from build123d import *

# Parameters (mm, degrees)
SKETCH2_R           = 2.168725958
SKETCH2_R_2         = 2.299626563
SKETCH2_R_3         = 2.061813599
SKETCH2_R_4         = 2.159
BOSS_EXTRUDE1_DEPTH = 2.54
SKETCH3_W           = 2.54
SKETCH3_H           = 88.215633797
BOSS_EXTRUDE2_DEPTH = 17.78
SKETCH5_R           = 3.175
CUT_EXTRUDE2_DEPTH  = 17.78


with BuildPart() as part:
    # Sketch2 → Boss-Extrude1 (new body)
    with BuildSketch(Plane.XY):
        Polygon((33.041228817, 37.6809), (33.041228817, 9.671924958), (33.041228817, -38.409527683), (33.041228817, -46.223073917), (-33.041228817, -46.223073917), (-33.041228817, -38.409527683), (-33.041228817, 9.671924958), (-33.041228817, 37.6809), (-33.041228817, 41.99255988), (33.041228817, 41.99255988), align=None)
        with Locations((19.8374, -24.8158)):
            Circle(SKETCH2_R, mode=Mode.SUBTRACT)
        with Locations((21.996003552, 27.558503658)):
            Circle(SKETCH2_R, mode=Mode.SUBTRACT)
        with Locations((-0.000312071, 34.695463786)):
            Circle(SKETCH2_R_2, mode=Mode.SUBTRACT)
        with Locations((-21.9964, 27.559)):
            Circle(SKETCH2_R_3, mode=Mode.SUBTRACT)
        with Locations((-19.8374, 14.859)):
            Circle(SKETCH2_R_4, mode=Mode.SUBTRACT)
        with Locations((-19.8374, -24.8158)):
            Circle(SKETCH2_R, mode=Mode.SUBTRACT)
        Polygon((15.652792396, 9.671924958), (15.652792396, 27.558503658), (-13.85744492, 27.558503658), (-15.780925581, 27.558503658), (-15.780925581, 9.671924958), (-15.780925581, -38.409527683), (15.652792396, -38.409527683), align=None, mode=Mode.SUBTRACT)
    extrude(amount=BOSS_EXTRUDE1_DEPTH)

    # Sketch3 → Boss-Extrude2 (add)
    with BuildSketch(Plane.XY.offset(2.54)):
        with Locations((-31.771228817, -2.115257018)):
            Rectangle(SKETCH3_W, SKETCH3_H)
    extrude(amount=BOSS_EXTRUDE2_DEPTH)

    # Sketch5 → Cut-Extrude2 (cut)
    with BuildSketch(Plane(origin=(-30.501228817, 0, 0), x_dir=(0, 0, -1), z_dir=(1, 0, 0))):
        with Locations((-11.43, -35.196119692)):
            Circle(SKETCH5_R)
        with Locations((-11.43, -13.142211243)):
            Circle(SKETCH5_R)
        with Locations((-11.43, 8.911697206)):
            Circle(SKETCH5_R)
        with Locations((-11.43, 30.965605655)):
            Circle(SKETCH5_R)
    extrude(amount=-CUT_EXTRUDE2_DEPTH, mode=Mode.SUBTRACT)


solid = part.part
Source: CAD feature listing. Evaluate the final solid. Frame: model axes, mm. A direction names the side the tool comes from. Give positions to 0.01 mm unless a question says otherwise; leave off trailing zeros. Write each loop counter-clockwise with the first axis right and the second up, starting at its lowest first coordinate (ties: lowest second). Pieces come first, ordered by that corner, then holes. Notation, with made-up numbers: (31.5, 41) -> (54.5, 41) arc R13 ccw to (54.5, 66) -> close; hole circle Ø11 at (8, 85.25). An arc over 180 degrees is marked (long way). Return JSON: item names as keys, results as strings. Group by question number.
1. Material intervals for line 1 (Y direction, x = -31.35, z = 11.43); line 2 (Y direction, x = 20, z = 2.25); line 3 (X direction, y = 25, z = 1.5), sorted ascending. Write a range as from..to.
2. Section C-C, the plane z = 11.43. Output: boundary loops of the cut face in (x, y).
3. Access query for faces 1 (the face through (33.041, -3, 1)), 2 (the face through (0, 27.559, 1)), 3 (the face through (16, -1, 2.54)). Directions: +Z, -Z, +X, -X, +Y, -Y. A direction counts if a zero-diameter tool reaches every point of the face in a straight line with its end or side. Return the directions, or none.
4. Section B-B, the plane x = -7.5. Output: boundary loops of the cut face in (y, z), then the cut area to 3 significant figures.
5. Section D-D, the plane x = 27. Output: boundary loops of the cut face in (y, z), then the cut area to 3 significant figures.
6. Mould query, pull axis Y, two halves, no side actions, for faces 4 (the face through (-33.041, -3, 10)), 5 (the face through (21.53, 25.44, 1.25)), 6 (the face through (-7, 41.993, 2)). Classes: +Y half, -Y half, draft (parallel to the pull), parting line (faces both ways), or undercut.
7. Section A-A, the plane y = 22. Output: boundary loops of the cut face in (x, z).
8. Pin query (flat end, axial travel): pin 1 Ø7.5 at (x, y) = (0, 34.7) entering from -Z; pin 2 Ø4 at (x, y) = (-19.84, -24.82) entering from -Z; pin 3 Ø2 at (x, y) = (22, -22.5) entering from +Z; pin 4 Ø7.5 at (y, z) = (8.91, 11.43) entering from +X. Return the tip coordinate at first contact, or that it passes through.
Determined:
{
 "1": {"line 1": "y = -46.22..-38.37, -32.02..-16.32, -9.97..5.74, 12.09..27.79, 34.14..41.99", "line 2": "y = -46.22..-26.98, -22.65..26.71, 28.41..41.99", "line 3": "x = -33.04..-15.78, 15.65..33.04"},
 "2": {"outline": "(-33.04, -46.22) -> (-30.5, -46.22) -> (-30.5, -38.37) -> (-33.04, -38.37) -> close; (-33.04, -32.02) -> (-30.5, -32.02) -> (-30.5, -16.32) -> (-33.04, -16.32) -> close; (-33.04, -9.97) -> (-30.5, -9.97) -> (-30.5, 5.74) -> (-33.04, 5.74) -> close; (-33.04, 12.09) -> (-30.5, 12.09) -> (-30.5, 27.79) -> (-33.04, 27.79) -> close; (-33.04, 34.14) -> (-30.5, 34.14) -> (-30.5, 41.99) -> (-33.04, 41.99) -> close"},
 "3": {"face 1": "+Z, -Z, +X, +Y, -Y", "face 2": "+Z, -Z", "face 3": "+Z, +X, +Y, -Y"},
 "4": {"outline": "(-46.22, 0) -> (-38.41, 0) -> (-38.41, 2.54) -> (-46.22, 2.54) -> close; (27.56, 0) -> (41.99, 0) -> (41.99, 2.54) -> (27.56, 2.54) -> close", "area": "56.5 mm2"},
 "5": {"outline": "(-46.22, 0) -> (41.99, 0) -> (41.99, 2.54) -> (-46.22, 2.54) -> close", "area": "224 mm2"},
 "6": {"face 4": "draft", "face 5": "undercut", "face 6": "+Y half"},
 "7": {"outline": "(-33.04, 0) -> (-15.78, 0) -> (-15.78, 2.54) -> (-30.5, 2.54) -> (-30.5, 20.32) -> (-33.04, 20.32) -> close; (15.65, 0) -> (33.04, 0) -> (33.04, 2.54) -> (15.65, 2.54) -> close"},
 "8": {"pin 1": "stops at z = 0", "pin 2": "passes through", "pin 3": "stops at z = 2.54", "pin 4": "stops at x = -30.5"}
}
